Design review of the part built by this model. Coordinates are the model's own, in mm. Face numbers are marked on the shaded views. A direction names the side the tool comes from. Coordinates: 2 decimals unless noted, no trailing zeros. Write each loop counter-clockwise with the first axis right and the second up, starting at its lowest first coordinate (ties: lowest second). Pieces come first, ordered by that corner, then holes. Notation, with made-up numbers: (84, 9.25) -> (129, 9.25) arc R20 cw to (129, 32.25) -> close; hole circle Ø7 at (30.25, 33.5). An arc over 180 degrees is marked (long way). One line per question, with ' | ' between items. Start each with the question number.
Q1. Draft analysis for pull direction Z (two halves, no side actions). For the marked faces 3, 4 and 5, state which applies: pulls with the +Z half, pulls with the -Z half, needs draft (parallel to the pull), parting line crosses it, or undercut.
Q2. For the marked faces 1 and 2, list the 3-axis set-ups (+Z, -Z, +X, -X, +Y, -Y) from which the entire face can be reached by the end or side of a thin tool; tool diameter is ignored.
Q3. Add section D-D on y = -5. State the section outline as (x, z) points.
Q4. For P1, Ø8, axis at x = -29.5, y = 37, coming from the -Z side (3 decimals); P2, Ø6, axis at x = 46.5, y = 54.5, coming from the -Z side; P3, Ø11, axis at x = 93, y = 51.5, coming from the -Z side, all flat-tipped, find the tip position at first contact; note any pin that passes through.
Q5. Wall thickness on probe 1 along Y at (x, z) = (60.5, 47.5); probe 2 along Y at (x, z) = (80, -12); probe 3 along Z at (x, y) = (5, 37.5): over which ranges is each line inside the solid? List them lowest first.
Q6. Add section B-B on z = -45.5. State the section outline as (x, y) points.
Q7. Add section A-A on y = 69.5. State the section outline as (x, z) points.
Q8. Add section C-C on x = -52.5. State the section outline as (y, z) points.
from build123d import *

# Parameters (mm, degrees)
SKETCH1_W                = 200
SKETCH1_H                = 150
BOSS_EXTRUDE1_DEPTH      = 15
SKETCH1_5_W              = 200
SKETCH1_5_H              = 10
REVOLVE1_ANGLE           = 90
BOSS_EXTRUDE3_REACH      = 197.256
BOSS_EXTRUDE3_END_RADIUS = 140
SKETCH1_6_W              = 10
SKETCH1_6_H              = 10
CUT_EXTRUDE1_DEPTH       = 130
CUT_EXTRUDE2_DEPTH       = 60
SKETCH7_W                = 10.545965087
SKETCH7_H                = 8.248079899
CUT_EXTRUDE5_DEPTH       = 74


with BuildPart() as part:
    # Sketch1 → Boss-Extrude1 (new body)
    with BuildSketch(Plane(origin=(0, 0, 0), x_dir=(1, 0, 0), z_dir=(0, 1, 0))):
        Rectangle(SKETCH1_W, SKETCH1_H)
    extrude(amount=-BOSS_EXTRUDE1_DEPTH)

    # Sketch1<5> → Revolve1 (revolve)
    with BuildSketch(Plane(origin=(0, 0, 0), x_dir=(1, 0, 0), z_dir=(0, 1, 0))):
        with Locations((0, 70)):
            Rectangle(SKETCH1_5_W, SKETCH1_5_H)
    revolve(axis=Axis((-100, 0, 75), (1, 0, 0)), revolution_arc=REVOLVE1_ANGLE)

    # Boss-Extrude3: up to this cylinder (the profile starts inside it)
    boss_extrude3_end = Plane(origin=(0, 0, 75), z_dir=(-1, 0, 0)) * Cylinder(BOSS_EXTRUDE3_END_RADIUS, 865.512, mode=Mode.PRIVATE)
    # Sketch1<6> → Boss-Extrude3 (add, up to the surface)
    with BuildSketch(Plane(origin=(0, 0, 0), x_dir=(1, 0, 0), z_dir=(0, 1, 0)), mode=Mode.PRIVATE) as boss_extrude3_sk1:
        with Locations((-95, -70)):
            Rectangle(SKETCH1_6_W, SKETCH1_6_H)
    boss_extrude3_tool1 = extrude(boss_extrude3_sk1.sketch, amount=BOSS_EXTRUDE3_REACH, mode=Mode.PRIVATE) & boss_extrude3_end
    add(boss_extrude3_tool1.solids().sort_by_distance((-95, 0, 70))[0])
    # Sketch1<6> → Boss-Extrude3 (add, up to the surface)
    with BuildSketch(Plane(origin=(0, 0, 0), x_dir=(1, 0, 0), z_dir=(0, 1, 0)), mode=Mode.PRIVATE) as boss_extrude3_sk2:
        with Locations((95, -70)):
            Rectangle(SKETCH1_6_W, SKETCH1_6_H)
    boss_extrude3_tool2 = extrude(boss_extrude3_sk2.sketch, amount=BOSS_EXTRUDE3_REACH, mode=Mode.PRIVATE) & boss_extrude3_end
    add(boss_extrude3_tool2.solids().sort_by_distance((95, 0, 70))[0])

    # Sketch4 → Cut-Extrude1 (cut)
    with BuildSketch(Plane.XY.offset(65)):
        Polygon((-100, -10), (90, 0), (-100, 0), align=None)
    extrude(amount=-CUT_EXTRUDE1_DEPTH, mode=Mode.SUBTRACT)

    # Sketch5 → Cut-Extrude2 (cut)
    with BuildSketch(Plane.ZY.offset(80)):
        Polygon((66.095917942, 143.620915339), (26.904082058, 135.620915339), (21.904082058, 160.115812766), (61.095917942, 168.115812766), align=None)
    extrude(amount=-CUT_EXTRUDE2_DEPTH, mode=Mode.SUBTRACT)

    # Sketch7 → Cut-Extrude5 (cut)
    with BuildSketch(Plane.ZY.offset(80)):
        with Locations((59.727017457, 145.87596005)):
            Rectangle(SKETCH7_W, SKETCH7_H)
    extrude(amount=CUT_EXTRUDE5_DEPTH, mode=Mode.SUBTRACT)


solid = part.part
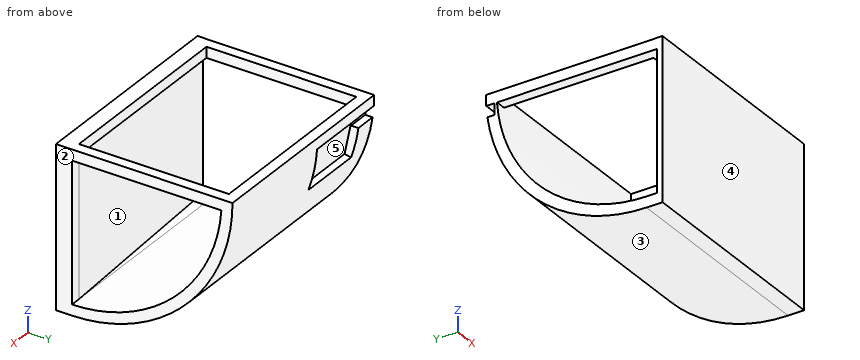
Output values:
1) face 3: pulls with the -Z half | face 4: needs draft | face 5: undercut
2) face 1: -X | face 2: +Z, -Z, +X, +Y, -Y
3) outline: (-100, -75) -> (100, -75) -> (100, 75) -> (-100, 75) -> (-100, 65) -> (-5, 65) -> (-5, -65) -> (-100, -65) -> close
4) P1: stops at z = -71.325 | P2: stops at z = -65.88 | P3: stops at z = -67.77
5) probe 1: y = -15 to -1.55, 137.27 to 147.46 | probe 2: y = -15 to -0.53, 109.69 to 122.19 | probe 3: z = -70.24 to -59.88
6) outline: (-100, -15) -> (100, -15) -> (100, 0) -> (90, 0) -> (-100, -10) -> close; (-100, 71.27) -> (100, 71.27) -> (100, 89.33) -> (-100, 89.33) -> close
7) outline: (-100, -57.93) -> (100, -57.93) -> (100, -46.53) -> (-100, -46.53) -> close; (-100, 65) -> (-90, 65) -> (-90, 75) -> (-100, 75) -> close; (90, 65) -> (100, 65) -> (100, 75) -> (90, 75) -> close
8) outline: (-15, -75) -> (0, -75) arc R150 ccw to (141.66, 25.67) -> (135.62, 26.9) -> (143.62, 66.1) -> (149.66, 64.86) arc R150 ccw to (150, 75) -> (140, 75) arc R140 cw to (0, -65) -> (-7.5, -65) -> (-7.5, 65) -> (0, 65) -> (0, 75) -> (-15, 75) -> close
